Design review of the part built by this model. Coordinates are the model's own, in mm. A direction names the side the tool comes from. Coordinates: 2 decimals unless noted, no trailing zeros. Loops run counter-clockwise (first coordinate to the right, second up) from the corner with the lowest first, then second, coordinate; pieces in that order, holes last. Notation, with made-up numbers: (-22.5, 28) -> (-4.5, 28) arc R20 ccw to (-4.5, 63) -> close; hole circle Ø2 at (-5, 69). An arc over 180 degrees is marked (long way). Use CSV: the item, a comma, the result in double quotes.
```python
from build123d import *

# Parameters (mm, degrees)
SCHIZZO1_R                   = 2
ESTRUSIONE_ESTRUSIONE1_DEPTH = 2.5
ESTRUSIONE_ESTRUSIONE2_DEPTH = 7.5
TAGLIO_ESTRUSIONE1_DEPTH     = 55.551477823
ESTRUSIONE_ESTRUSIONE3_DEPTH = 4.632546


with BuildPart() as part:
    # Schizzo1 → Estrusione-Estrusione1 (new body)
    with BuildSketch(Plane.XY):
        with BuildLine():
            Line((0, -6), (43.5, -6))
            Line((43.5, -6), (59.085369345, 3.967259523))
            Line((59.085369345, 3.967259523), (56.58948898, 7.869958879))
            Line((56.58948898, 7.869958879), (43.5, -0.501118559))
            Line((43.5, -0.501118559), (0, 6))
            ThreePointArc((0, 6), (-6, 0), (0, -6))
        make_face()
        Circle(SCHIZZO1_R, mode=Mode.SUBTRACT)
        with Locations((12, -0.8)):
            Circle(SCHIZZO1_R, mode=Mode.SUBTRACT)
    extrude(amount=ESTRUSIONE_ESTRUSIONE1_DEPTH)

    # Schizzo3 → Estrusione-Estrusione2 (add)
    with BuildSketch(Plane(origin=(0, 0, 0), x_dir=(-1, 0, 0), z_dir=(0, 0, -1))):
        Polygon((-56.58948898, 7.869958879), (-59.085369345, 3.967259523), (-56.979238352, 2.62033256), (-54.483357987, 6.523031917), align=None)
    extrude(amount=ESTRUSIONE_ESTRUSIONE2_DEPTH)

    # Schizzo4 → Taglio-Estrusione1 (cut, through all)
    with BuildSketch(Plane(origin=(12.854369278, -20.099817049, 0), x_dir=(0.8424523970071469, 0.5387707850068642, 0), z_dir=(-0.5387707850068642, 0.8424523970071469, 0))):
        with BuildLine():
            Line((51.91405456, 0.5), (51.91405456, -2.5))
            Line((51.91405456, -2.5), (48.91405456, -2.5))
            ThreePointArc((48.91405456, -2.5), (51.035374903, -1.621320344), (51.91405456, 0.5))
        make_face()
    extrude(amount=-TAGLIO_ESTRUSIONE1_DEPTH, mode=Mode.SUBTRACT)

    # Schizzo5 → Estrusione-Estrusione3 (add)
    with BuildSketch(Plane(origin=(12.854369278, -20.099817049, 0), x_dir=(0.8424523970071469, 0.5387707850068642, 0), z_dir=(-0.5387707850068642, 0.8424523970071469, 0))):
        with BuildLine():
            Line((49.41405456, 1), (49.41405456, 0))
            Line((49.41405456, 0), (48.41405456, 0))
            ThreePointArc((48.41405456, 0), (49.121161341, 0.292893219), (49.41405456, 1))
        make_face()
    extrude(amount=-ESTRUSIONE_ESTRUSIONE3_DEPTH)

    # Specchia4: part across plane


with BuildPart() as part_1:
    add(part.part)
    add(part.part.mirror(Plane.XY.offset(-7.5)))


solid = part_1.part
```
Item 1: Add section C-C (x = 12). Give the boundary of the cut face in (y, z), then the cut area to 3 significant figures.
Checked values:
outline,"(-6, -17.5) -> (-2.8, -17.5) -> (-2.8, -15) -> (-6, -15) -> close; (-6, 0) -> (-2.8, 0) -> (-2.8, 2.5) -> (-6, 2.5) -> close; (1.2, -17.5) -> (4.21, -17.5) -> (4.21, -15) -> (1.2, -15) -> close; (1.2, 0) -> (4.21, 0) -> (4.21, 2.5) -> (1.2, 2.5) -> close"
area,"31.0 mm^2"
Item 2: Add section B-B (y = -5). Give the boundary of the cut face in (x, z).
Checked values:
outline,"(-3.32, -17.5) -> (45.06, -17.5) -> (45.06, -15) -> (-3.32, -15) -> close; (-3.32, 0) -> (45.06, 0) -> (45.06, 2.5) -> (-3.32, 2.5) -> close"
Item 3: Clearance check with flat-ended pins moving along their axes: pin 1 (1.5 mm diameter, centred on y = 2.5, z = -10.5, fed in from +X); pin 2 (3 mm diameter, centred on x = 29, z = -12, fed in from -Y); pin 3 (6 mm diameter, centred on x = 5.5, z = -2, fed in from +Y). State where each tip first meets the part, or that it passes through.
Checked values:
pin 1,"x = 57.96"
pin 2,"through"
pin 3,"y = 5.51"
Item 4: Machinability: for faces 4 (the face through (22.054, 2.704, 1.232)), 5 (the face through (18, -1, -17.5)), 6 (the face through (55.75, 4.54, -7.59)), which of the approach directions +Z, -Z, +X, -X, +Y, -Y give a long, thin tool a straight path to every point of the face, cutting with its end or side? Answer none if there is none.
Checked values:
face 4,"+Z, -Z, +Y"
face 5,"-Z, +X, -X, +Y, -Y"
face 6,"-X, -Y"
Item 5: Draft analysis for pull direction X (two halves, no side actions). For faces 1 (the face through (10.002, -0.712, 1.232)), 2 (the face through (21, -6, -16)), 3 (the face through (57.06, 5.46, -16.645)), state which applies: pulls with the +X half, pulls with the -X half, needs draft (parallel to the pull), parting line crosses it, or undercut.
Checked values:
face 1,"undercut"
face 2,"needs draft"
face 3,"pulls with the +X half"
Item 6: Add section A-A (x = 3.5). Give the boundary of the cut face in (y, z), then the cut area to 3 significant figures.
Checked values:
outline,"(-6, -17.5) -> (5.48, -17.5) -> (5.48, -15) -> (-6, -15) -> close; (-6, 0) -> (5.48, 0) -> (5.48, 2.5) -> (-6, 2.5) -> close"
area,"57.4 mm^2"
Item 7: Add section D-D (z = -5.5). Give the boundary of the cut face in (x, y).
Checked values:
outline,"(54.48, 6.52) -> (56.98, 2.62) -> (59.09, 3.97) -> (56.59, 7.87) -> close"
Item 8: To check wall thickness, follow line 1 along Z through (x, y) = (20.5, 2.75); line 2 along X through (y, z) = (-1, 1.25); line 3 along Y through (x, z) = (0, 1.95). State the ranges of each line that lie inside material, in increasing order.
Checked values:
line 1,"-17.5 to -15, 0 to 2.5"
line 2,"-5.92 to -1.73, 1.73 to 10.01, 13.99 to 51.32"
line 3,"-6 to -2, 2 to 6"
